from build123d import *

# Parameters (mm, degrees)
PAD_DEPTH    = 30
SKETCH001_W  = 9.2
SKETCH001_H  = 15
PAD001_DEPTH = 2


with BuildPart() as part:
    # Sketch → Pad (new body)
    with BuildSketch(Plane.XY):
        Polygon((-10.883168, 0.282843), (29.116832, 0.282843), (29.116832, 15.282843), align=None)
    extrude(amount=PAD_DEPTH)

    # Sketch001 → Pad001 (new body)
    with BuildSketch(Plane.XZ.offset(-0.282843)):
        with Locations((3.672524, 15)):
            Rectangle(SKETCH001_W, SKETCH001_H)
        with Locations((20.872524, 15)):
            Rectangle(SKETCH001_W, SKETCH001_H)
    extrude(amount=PAD001_DEPTH)


solid = part.part
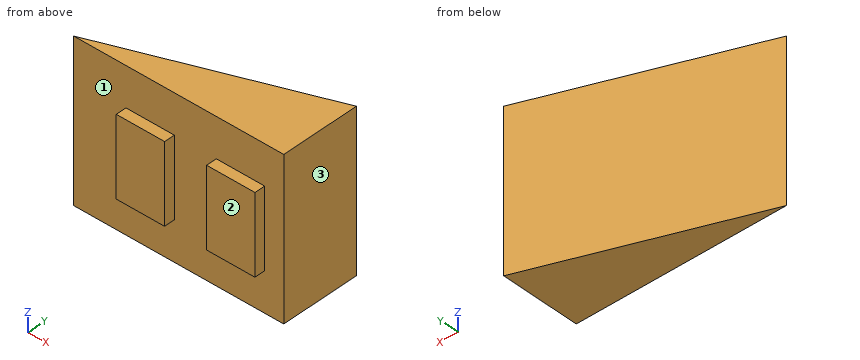
The model under review builds one solid part; all positions refer to its coordinate system, in mm. Face numbers are marked on the shaded views. Round coordinates to 2 decimals unless told otherwise and drop trailing zeros. Write each loop counter-clockwise with the first axis right and the second up, starting at its lowest first coordinate (ties: lowest second). Pieces come first, ordered by that corner, then holes. Notation, with made-up numbers: (63.5, 11.5) - (99.5, 11.5) arc R17 cw to (99.5, 23.5) - close; hole circle Ø4 at (7, 75). An arc over 180 degrees is marked (long way). One line per item, written item: value. Start each with the question number.
1. Consider section C-C on y = 8. Write out the cut boundary in (x, z), and give its area (3 significant figures).
2. Consider section B-B on x = 4.5. Write out the cut boundary in (y, z), and give its area (3 significant figures).
3. Consider section A-A on z = 16. Write out the cut boundary in (x, y), and give its area (3 significant figures).
4. Consider section D-D on z = 6.5. Write out the cut boundary in (x, y).
5. To check wall thickness, follow L1, parallel to X at y = -0.5, z = 21.25; L2, parallel to Y at x = 24, z = 18.75; L3, parallel to Y at x = -1.5, z = 2. State the ranges of each line that lie inside material, in increasing order. Write a range as from..to.
6. The part is to be moulded in two halves that separate along X. For the marked faces 1, 2 and 3, say which applies: released by +X, released by -X, zero draft, split by the parting line, or undercut.
7. Clearance check with flat-ended pins moving along their axes: P1, Ø5, axis at x = 2.5, y = 9.5, coming from the +Z side; P2, Ø1.6, axis at y = -1, z = 12, coming from the -X side; P3, Ø1.5, axis at x = -6, z = 26.5, coming from the +Y side; P4, Ø6, axis at x = 10.5, z = 15.5, coming from the +Y side. State where each tip first meets the part, or that it passes through.
Checks:
1. outline: (9.7, 0) - (29.12, 0) - (29.12, 30) - (9.7, 30) - close
1. area: 583 mm^2
2. outline: (-1.72, 7.5) - (0.28, 7.5) - (0.28, 0) - (6.05, 0) - (6.05, 30) - (0.28, 30) - (0.28, 22.5) - (-1.72, 22.5) - close
2. area: 203 mm^2
3. outline: (-10.88, 0.28) - (-0.93, 0.28) - (-0.93, -1.72) - (8.27, -1.72) - (8.27, 0.28) - (16.27, 0.28) - (16.27, -1.72) - (25.47, -1.72) - (25.47, 0.28) - (29.12, 0.28) - (29.12, 15.28) - close
3. area: 337 mm^2
4. outline: (-10.88, 0.28) - (29.12, 0.28) - (29.12, 15.28) - close
5. L1: x = -0.93..8.27, 16.27..25.47
5. L2: y = -1.72..13.36
5. L3: y = 0.28..3.8
6. face 1: undercut
6. face 2: zero draft
6. face 3: released by +X
7. P1: passes through
7. P2: stops at x = -0.93
7. P3: stops at y = 2.4
7. P4: stops at y = 9.43
